Geometry: final body of the model. Coordinates: model frame, mm. A direction names the side the tool comes from. Give positions to 0.01 mm unless a question says otherwise; leave off trailing zeros. Loops run counter-clockwise (first coordinate to the right, second up) from the corner with the lowest first, then second, coordinate; pieces in that order, holes last.
```python
from build123d import *

# Parameters (mm, degrees)
SKETCH1_R                 = 13.85
BOSS_EXTRUDE1_DEPTH       = 19
SKETCH2_R                 = 2.5
BOSS_EXTRUDE2_DEPTH       = 14
M3X0_5_TAPPED_HOLE1_D     = 2.5
M3X0_5_TAPPED_HOLE1_DEPTH = 7.5
M3X0_5_TAPPED_HOLE1_TIP   = 0.751075774


with BuildPart() as part:
    # Sketch1 → Boss-Extrude1 (new body)
    with BuildSketch(Plane(origin=(0, 0, 0), x_dir=(1, 0, 0), z_dir=(0, 1, 0))):
        Circle(SKETCH1_R)
    extrude(amount=BOSS_EXTRUDE1_DEPTH)

    # Sketch2 → Boss-Extrude2 (add)
    with BuildSketch(Plane(origin=(0, 19, 0), x_dir=(1, 0, 0), z_dir=(0, 1, 0))):
        Circle(SKETCH2_R)
    extrude(amount=BOSS_EXTRUDE2_DEPTH)

    # M3x0.5 Tapped Hole1
    with Locations(Plane(origin=(0, 0, 0), x_dir=(-1, 0, 0), z_dir=(0, -1, 0))):
        with Locations((0, -8), (9.5, 0), (0, 8), (-9.5, 0)):
            Hole(M3X0_5_TAPPED_HOLE1_D / 2, depth=M3X0_5_TAPPED_HOLE1_DEPTH)
            with Locations((0, 0, -(M3X0_5_TAPPED_HOLE1_DEPTH + M3X0_5_TAPPED_HOLE1_TIP / 2))):  # 118° drill point
                Cone(0, M3X0_5_TAPPED_HOLE1_D / 2, M3X0_5_TAPPED_HOLE1_TIP, mode=Mode.SUBTRACT)


solid = part.part
```
Q1. Section query A-A, the plane y = 7. Return loops of the section in (x, z), and give its area (3 significant figures).
Q2. Mould query, pull axis Z, two halves, no side actions, for faces 4 (the face through (13.21, 9.37, -4.16)), 5 (the face through (-0.27, 3.8, -6.78)), 6 (the face through (0, 19, 3)). Classes: +Z half, -Z half, draft (parallel to the pull), parting line (faces both ways), or undercut.
Q3. Section query D-D, the plane x = -5.25. Return loops of the section in (y, z), and give its area (3 significant figures).
Q4. Pin query (flat end, axial travel): pin 1 Ø2 at (y, z) = (4.5, -3.5) entering from -X; pin 2 Ø3 at (y, z) = (17, -3.5) entering from -X; pin 3 Ø1.5 at (y, z) = (19.5, -10) entering from +X. Return the tip coordinate at first contact, or that it passes through.
Q5. Reachability of faces 1 (the face through (0, 0, 0)), 2 (the face through (-0.54, 25.9, 2.44)), 3 (the face through (8.25, 3.8, -0.05)) from +Z, -Z, +X, -X, +Y, -Y: full face, straight path, thin tool, end or side. Return the list, or none.
Q6. Material intervals for probe 1 along Z at (x, y) = (0, 5.25); probe 2 along Z at (x, y) = (-0.5, 4); probe 3 along Y at (x, z) = (8.5, 4.75), sorted ascending.
Q7. Section query C-C, the plane z = -4.5. Return loops of the section in (x, y), and give its area (3 significant figures).
Q8. Section query B-B, the plane y = 16. Return loops of the section in (x, z).
Resolved:
1. outline: circle Ø27.7 at (0, 0); hole circle Ø2.5 at (-9.5, 0); hole circle Ø2.5 at (0, -8); hole circle Ø2.5 at (0, 8); hole circle Ø2.5 at (9.5, 0)
1. area: 583 mm2
2. face 4: parting line
2. face 5: undercut
2. face 6: draft
3. outline: (0, -12.82) - (19, -12.82) - (19, 12.82) - (0, 12.82) - close
3. area: 487 mm2
4. pin 1: stops at x = -13.62
4. pin 2: stops at x = -13.7
4. pin 3: stops at x = 10.13
5. face 1: +Z, -Z, +X, -X, -Y
5. face 2: +Y
5. face 3: -Y
6. probe 1: z = -13.85 to -9.25, -6.75 to 6.75, 9.25 to 13.85
6. probe 2: z = -13.84 to -9.15, -6.85 to 6.85, 9.15 to 13.84
6. probe 3: y = 0 to 19
7. outline: (-13.1, 0) - (13.1, 0) - (13.1, 19) - (-13.1, 19) - close
7. area: 498 mm2
8. outline: circle Ø27.7 at (0, 0)
